```python
from build123d import *
from build123d.topology import SkipClean

# Parameters (mm, degrees)
SKETCH_1_W          = 50
SKETCH_1_H          = 50
SKETCH_1_R          = 21.5
SKETCH_1_R_2        = 13.5
SKETCH_1_R_3        = 1.5
EXTRUDE_1_DEPTH     = 8
SKETCH_2_R          = 21.5
CUT_EXTRUDE_1_DEPTH = 6
SKETCH_3_W          = 50
SKETCH_3_H          = 5
CUT_EXTRUDE_2_DEPTH = 27
CUT_EXTRUDE_3_DEPTH = 10
SKETCH_5_W          = 59.949446365
SKETCH_5_H          = 15
CUT_EXTRUDE_4_DEPTH = 6
SKETCH_6_R          = 13.5
CUT_EXTRUDE_5_DEPTH = 10
SKETCH_7_W          = 38
SKETCH_7_H          = 25.671468353
CUT_EXTRUDE_6_DEPTH = 6
EXTRUDE_START       = 6
EXTRUDE_2_DEPTH     = 6
SKETCH_9_R          = 1.25
CUT_EXTRUDE_7_DEPTH = 5
FILLET_1_R          = 1
FILLET_2_R          = 3
CHAMFER_1_SIZE      = 3
CUT_EXTRUDE_8_DEPTH = 51
CUT_EXTRUDE_9_DEPTH = 38


with BuildPart() as part:
    # 草图1 → 凸台-拉伸1 (new body)
    # profile 1 of 3: a face of its own
    with BuildSketch(Plane.XY):
        Rectangle(SKETCH_1_W, SKETCH_1_H)
        Circle(SKETCH_1_R, mode=Mode.SUBTRACT)
    # profile 2 of 3: a face of its own
    with BuildSketch(Plane.XY):
        Circle(SKETCH_1_R)
        Circle(SKETCH_1_R_2, mode=Mode.SUBTRACT)
        with Locations((0, 17.5)):
            Circle(SKETCH_1_R_3, mode=Mode.SUBTRACT)
        with Locations((12.374368671, 12.374368671)):
            Circle(SKETCH_1_R_3, mode=Mode.SUBTRACT)
        with Locations((17.5, 0)):
            Circle(SKETCH_1_R_3, mode=Mode.SUBTRACT)
        with Locations((12.374368671, -12.374368671)):
            Circle(SKETCH_1_R_3, mode=Mode.SUBTRACT)
        with Locations((0, -17.5)):
            Circle(SKETCH_1_R_3, mode=Mode.SUBTRACT)
        with Locations((-12.374368671, -12.374368671)):
            Circle(SKETCH_1_R_3, mode=Mode.SUBTRACT)
        with Locations((-17.5, 0)):
            Circle(SKETCH_1_R_3, mode=Mode.SUBTRACT)
        with Locations((-12.374368671, 12.374368671)):
            Circle(SKETCH_1_R_3, mode=Mode.SUBTRACT)
    # profile 3 of 3: a face of its own
    with BuildSketch(Plane.XY):
        Circle(SKETCH_1_R_2)
    extrude(amount=EXTRUDE_1_DEPTH)

    # 草图2 → 切除-拉伸1 (cut)
    with BuildSketch(Plane.XY.offset(8)):
        Circle(SKETCH_2_R)
    extrude(amount=-CUT_EXTRUDE_1_DEPTH, mode=Mode.SUBTRACT)

    # 草图3 → 切除-拉伸2 (cut)
    with BuildSketch(Plane.XY.offset(8)):
        with Locations((0, 22.5)):
            Rectangle(SKETCH_3_W, SKETCH_3_H)
    extrude(amount=-CUT_EXTRUDE_2_DEPTH, mode=Mode.SUBTRACT)

    # 草图4 → 切除-拉伸3 (cut)
    with BuildSketch(Plane.XY.offset(8)):
        Polygon((-25, 5), (-25, 20), (-10, 20), align=None)
        Polygon((10, 20), (25, 5), (25, 20), align=None)
    extrude(amount=-CUT_EXTRUDE_3_DEPTH, mode=Mode.SUBTRACT)

    # 草图5 → 切除-拉伸4 (cut)
    with BuildSketch(Plane.XY.offset(8)):
        with Locations((-0.284795469, 12.5)):
            Rectangle(SKETCH_5_W, SKETCH_5_H)
    extrude(amount=-CUT_EXTRUDE_4_DEPTH, mode=Mode.SUBTRACT)

    # 草图6 → 切除-拉伸5 (cut)
    with BuildSketch(Plane.XY.offset(2)):
        Circle(SKETCH_6_R)
    extrude(amount=-CUT_EXTRUDE_5_DEPTH, mode=Mode.SUBTRACT)

    # 草图7 → 切除-拉伸6 (cut)
    with BuildSketch(Plane.XY.offset(8)):
        with Locations((0, -22.898040076)):
            Rectangle(SKETCH_7_W, SKETCH_7_H)
    extrude(amount=-CUT_EXTRUDE_6_DEPTH, mode=Mode.SUBTRACT)

    # 草图8 → 凸台-拉伸2 (add)
    with BuildSketch(Plane.XY.offset(8).offset(EXTRUDE_START)):
        with BuildLine():
            Line((19, -10.062305899), (19, -25))
            Line((19, -25), (25, -25))
            Line((25, -25), (25, 5))
            Line((25, 5), (20.910523666, 5))
            ThreePointArc((20.910523666, 5), (21.329105457, -2.70541317), (19, -10.062305899))
        make_face()
        with BuildLine():
            Line((-19, -25), (-19, -10.062305899))
            ThreePointArc((-19, -10.062305899), (-21.329105457, -2.70541317), (-20.910523666, 5))
            Line((-20.910523666, 5), (-25, 5))
            Line((-25, 5), (-25, -25))
            Line((-25, -25), (-19, -25))
        make_face()
    extrude(amount=-EXTRUDE_2_DEPTH)

    # 草图9 → 切除-拉伸7 (cut)
    with SkipClean():  # the faces are left unmerged after this step: merging them gives an invalid solid
        with BuildSketch(Plane(origin=(25, 0, 0), x_dir=(0, 0, -1), z_dir=(1, 0, 0))):
            with Locations(Location((-3.5, -16, 0), (0, 0, 90))):
                Circle(SKETCH_9_R)
            with Locations(Location((-3.5, -22, 0), (0, 0, 90))):
                Circle(SKETCH_9_R)
            with Locations(Location((-10.5, -16, 0), (0, 0, 90))):
                Circle(SKETCH_9_R)
            with Locations(Location((-10.5, -22, 0), (0, 0, 90))):
                Circle(SKETCH_9_R)
        cut_extrude_7 = extrude(amount=-CUT_EXTRUDE_7_DEPTH, mode=Mode.SUBTRACT)

    # 镜向1: 切除-拉伸7 across plane
    with SkipClean():  # the faces are left unmerged after this step: merging them gives an invalid solid
        add(cut_extrude_7.mirror(Plane(origin=(0, 0, 0), x_dir=(0, 0, 1), z_dir=(1, 0, 0))), mode=Mode.SUBTRACT)

    # 圆角1
    fillet_1_edges = [part.edges().sort_by_distance(p)[0] for p in [
        (20.910523666, 5, 8),
        (-20.910523666, 5, 11),
        (19, -10.062305899, 8),
        (-19, -10.062305899, 5),
    ]]
    fillet(fillet_1_edges, radius=FILLET_1_R)

    # 圆角2
    fillet_2_edges = [part.edges().sort_by_distance(p)[0] for p in [
        (10, 20, 1),
        (-10, 20, 1),
    ]]
    fillet(fillet_2_edges, radius=FILLET_2_R)

    # 倒角1
    chamfer_1_edges = [part.edges().sort_by_distance(p)[0] for p in [
        (22, -25, 14),
        (-22, -25, 14),
    ]]
    chamfer(chamfer_1_edges, length=CHAMFER_1_SIZE)

    # 草图10 → 切除-拉伸8 (cut)
    with BuildSketch(Plane(origin=(25, 0, 0), x_dir=(0, 0, -1), z_dir=(1, 0, 0))):
        Polygon((-2, -25), (0, -25), (0, -20), align=None)
    extrude(amount=-CUT_EXTRUDE_8_DEPTH, mode=Mode.SUBTRACT)

    # 草图11 → 切除-拉伸9 (cut)
    with BuildSketch(Plane.ZY.offset(-19)):
        Polygon((2, -25), (2, -20), (0, -20), align=None)
    extrude(amount=CUT_EXTRUDE_9_DEPTH, mode=Mode.SUBTRACT)


solid = part.part
```
Can you work these out from the model? Positions are in its coordinate system, mm. A direction names the side the tool comes from. Round coordinates to 2 decimals unless told otherwise and drop trailing zeros. Loops run counter-clockwise (first coordinate to the right, second up) from the corner with the lowest first, then second, coordinate; pieces in that order, holes last. Notation, with made-up numbers: M 9,36.5 L 59,36.5 A23 cw 59,54.5 Z; hole C 66.25,19.25 d10. An arc over 180 degrees is marked long. Answer as a JSON object with one key per item and string values. Group by question number.
Q1. On a 3-axis mill with a long thin cutter (end or side, diameter ignored), from which of +Z, -Z, +X, -X, +Y, -Y can I reach the whole of each face in a straight line? I mean faces 1 (the cylindrical face through (22.535, -21.328, 11.554)), 2 (the cylindrical face through (-22.54, -17.25, 3.55)), 3 (the flat face through (0, -20, 1)). Say none if no direction works.
Q2. Will these pins go through, and if not, where does the flat tip stop? pin 1 (2 mm diameter, centred on y = -16, z = 3.5, fed in from -X); pin 2 (3.5 mm diameter, centred on x = 12.37, y = -12.37, fed in from +Z); pin 3 (1.2 mm diameter, centred on y = -22, z = 3, fed in from +X).
Q3. Imagine slicing it at C-C, the plane x = 0. Please give me the cut outline in (y, z), then the cut area to 3 significant figures.
Q4. Imagine slicing it at B-B, the plane x = 17.5. Please give me the cut outline in (y, z).
Q5. We'd pull the mould along X, two halves only. Please class faces 4 (the cylindrical face through (16, 0, 1)), 5 (the flat face through (20, -22, 11)), 6 (the flat face through (-20, -22, 11)): +X half, -X half, draft (parallel to the pull), parting line (faces both ways), or undercut.
Q6. Please list where these lines run through material, in increasing order: L1, parallel to Y at x = 0, z = 0.55; L2, parallel to X at y = -0.5, z = 6.75; L3, parallel to X at y = -11, z = 4.5.
Q7. Imagine slicing it at A-A, the plane y = 17.5. Please give me the cut outline in (x, z).
Findings:
{
 "1": {"face 1": "+X", "face 2": "-X", "face 3": "+Z, -Z, -Y"},
 "2": {"pin 1": "stops at x = -20", "pin 2": "stops at z = 2", "pin 3": "stops at x = 20"},
 "3": {"outline": "M -20,0 L -19,0 L -19,2 L -20,2 Z; M -16,0 L -13.5,0 L -13.5,2 L -16,2 Z; M 13.5,0 L 16,0 L 16,2 L 13.5,2 Z; M 19,0 L 20,0 L 20,2 L 19,2 Z", "area": "14.0 mm2"},
 "4": {"outline": "M -20,0 L -1.5,0 L -1.5,2 L -20,2 Z; M 1.5,0 L 12.5,0 L 12.5,2 L 1.5,2 Z"},
 "5": {"face 4": "undercut", "face 5": "+X half", "face 6": "-X half"},
 "6": {"L1": "y = -20 to -19, -16 to -13.5, 13.5 to 16, 19 to 20", "L2": "x = -25 to -21.49, 21.49 to 25", "L3": "x = -25 to -19, 19 to 25"},
 "7": {"outline": "M -12.5,0 L -1.5,0 L -1.5,2 L -12.5,2 Z; M 1.5,0 L 12.5,0 L 12.5,2 L 1.5,2 Z"}
}
